Here's how the part is built. I have some questions about the finished solid (model axes, mm). A direction names the side the tool comes from. Round coordinates to 2 decimals unless told otherwise and drop trailing zeros. Order: outer loops, then holes, each group sorted by start corner. A loop starts at its lowest first (then second) coordinate and runs counter-clockwise, first axis right, second up. Notation, with made-up numbers: (-38.5, 76) -> (-13.5, 76) arc R16 ccw to (-13.5, 82) -> close; hole circle Ø11 at (24.5, 50). An arc over 180 degrees is marked (long way). Use a Markdown table: item, result. Add a question column.
from build123d import *

# Parameters (mm, degrees)
SKETCH1_W           = 8.25
SKETCH1_H           = 2.1
SKETCH1_H_2         = 20.8
SKETCH1_R           = 2.275
BOSS_EXTRUDE1_DEPTH = 28.45
BOSS_EXTRUDE2_START = -28.45
SKETCH1_4_W         = 8.25
SKETCH1_4_H         = 2.1
SKETCH1_4_H_2       = 20.8
SKETCH1_4_R         = 2.275
SKETCH1_4_W_2       = 40.9
SKETCH1_4_W_3       = 0.2
SKETCH1_4_W_4       = 8.45
SKETCH1_4_R_2       = 1.7
BOSS_EXTRUDE2_DEPTH = 2
SKETCH1_5_W         = 69.95
SKETCH1_5_H         = 38
BOSS_EXTRUDE3_DEPTH = 30.45
SKETCH1_6_W         = 69.95
SKETCH1_6_H         = 38
BOSS_EXTRUDE4_DEPTH = 5


with BuildPart() as part:
    # Sketch1 → Boss-Extrude1 (new body)
    # profile 1 of 5: a face of its own
    with BuildSketch(Plane.XY):
        Polygon((-28.9, 12.5), (-20.65, 12.5), (-9.8, 12.5), (-9.8, 23.6), (-28.9, 23.6), align=None)
    # profile 2 of 5: a face of its own
    with BuildSketch(Plane.XY):
        with Locations((-24.775, 11.45)):
            Rectangle(SKETCH1_W, SKETCH1_H)
    # profile 3 of 5: a face of its own
    with BuildSketch(Plane.XY):
        with Locations((-24.775, 0)):
            Rectangle(SKETCH1_W, SKETCH1_H_2)
        with Locations((-24.55, -4.85)):
            Circle(SKETCH1_R, mode=Mode.SUBTRACT)
        with Locations((-24.55, 4.85)):
            Circle(SKETCH1_R, mode=Mode.SUBTRACT)
    # profile 4 of 5: a face of its own
    with BuildSketch(Plane.XY):
        Polygon((9.8, 12.5), (20.45, 12.5), (28.9, 12.5), (37.05, 12.5), (37.05, 23.6), (9.8, 23.6), align=None)
    # profile 5 of 5: a face of its own
    with BuildSketch(Plane.XY):
        Polygon((28.9, 12.5), (28.9, 10.4), (28.9, -10.4), (37.05, -10.4), (37.05, 12.5), align=None)
        with Locations((32.55, -4.85)):
            Circle(SKETCH1_R, mode=Mode.SUBTRACT)
        with Locations((32.55, 4.85)):
            Circle(SKETCH1_R, mode=Mode.SUBTRACT)
    extrude(amount=-BOSS_EXTRUDE1_DEPTH)

    # Sketch1<4> → Boss-Extrude2 (add)
    # profile 1 of 16: a face of its own
    with BuildSketch(Plane.XY.offset(BOSS_EXTRUDE2_START)):
        Polygon((-28.9, 12.5), (-20.65, 12.5), (-9.8, 12.5), (-9.8, 23.6), (-28.9, 23.6), align=None)
    # profile 2 of 16: a face of its own
    with BuildSketch(Plane.XY.offset(BOSS_EXTRUDE2_START)):
        Polygon((9.8, 12.5), (20.45, 12.5), (28.9, 12.5), (37.05, 12.5), (37.05, 23.6), (9.8, 23.6), align=None)
    # profile 3 of 16: a face of its own
    with BuildSketch(Plane.XY.offset(BOSS_EXTRUDE2_START)):
        Polygon((-20.65, 10.4), (-20.45, 10.4), (20.45, 10.4), (20.45, 12.5), (9.8, 12.5), (-9.8, 12.5), (-20.65, 12.5), align=None)
    # profile 4 of 16: a face of its own
    with BuildSketch(Plane.XY.offset(BOSS_EXTRUDE2_START)):
        with Locations((-24.775, 11.45)):
            Rectangle(SKETCH1_4_W, SKETCH1_4_H)
    # profile 5 of 16: a face of its own
    with BuildSketch(Plane.XY.offset(BOSS_EXTRUDE2_START)):
        with Locations((-24.775, 0)):
            Rectangle(SKETCH1_4_W, SKETCH1_4_H_2)
        with Locations((-24.55, -4.85)):
            Circle(SKETCH1_4_R, mode=Mode.SUBTRACT)
        with Locations((-24.55, 4.85)):
            Circle(SKETCH1_4_R, mode=Mode.SUBTRACT)
    # profile 6 of 16: a face of its own
    with BuildSketch(Plane.XY.offset(BOSS_EXTRUDE2_START)):
        with Locations((-24.55, 4.85)):
            Circle(SKETCH1_4_R)
    # profile 7 of 16: a face of its own
    with BuildSketch(Plane.XY.offset(BOSS_EXTRUDE2_START)):
        with Locations((-24.55, -4.85)):
            Circle(SKETCH1_4_R)
    # profile 8 of 16: a face of its own
    with BuildSketch(Plane.XY.offset(BOSS_EXTRUDE2_START)):
        Rectangle(SKETCH1_4_W_2, SKETCH1_4_H_2)
    # profile 9 of 16: a face of its own
    with BuildSketch(Plane.XY.offset(BOSS_EXTRUDE2_START)):
        with Locations((-20.55, 0)):
            Rectangle(SKETCH1_4_W_3, SKETCH1_4_H_2)
    # profile 10 of 16: a face of its own
    with BuildSketch(Plane.XY.offset(BOSS_EXTRUDE2_START)):
        with Locations((24.675, 0)):
            Rectangle(SKETCH1_4_W_4, SKETCH1_4_H_2)
        with Locations((24.55, -4.85)):
            Circle(SKETCH1_4_R_2, mode=Mode.SUBTRACT)
        with Locations((24.55, 4.85)):
            Circle(SKETCH1_4_R_2, mode=Mode.SUBTRACT)
    # profile 11 of 16: a face of its own
    with BuildSketch(Plane.XY.offset(BOSS_EXTRUDE2_START)):
        with Locations((24.55, 4.85)):
            Circle(SKETCH1_4_R_2)
    # profile 12 of 16: a face of its own
    with BuildSketch(Plane.XY.offset(BOSS_EXTRUDE2_START)):
        with Locations((24.55, -4.85)):
            Circle(SKETCH1_4_R_2)
    # profile 13 of 16: a face of its own
    with BuildSketch(Plane.XY.offset(BOSS_EXTRUDE2_START)):
        with Locations((24.675, 11.45)):
            Rectangle(SKETCH1_4_W_4, SKETCH1_4_H)
    # profile 14 of 16: a face of its own
    with BuildSketch(Plane.XY.offset(BOSS_EXTRUDE2_START)):
        Polygon((28.9, 12.5), (28.9, 10.4), (28.9, -10.4), (37.05, -10.4), (37.05, 12.5), align=None)
        with Locations((32.55, -4.85)):
            Circle(SKETCH1_4_R, mode=Mode.SUBTRACT)
        with Locations((32.55, 4.85)):
            Circle(SKETCH1_4_R, mode=Mode.SUBTRACT)
    # profile 15 of 16: a face of its own
    with BuildSketch(Plane.XY.offset(BOSS_EXTRUDE2_START)):
        with Locations((32.55, 4.85)):
            Circle(SKETCH1_4_R)
    # profile 16 of 16: a face of its own
    with BuildSketch(Plane.XY.offset(BOSS_EXTRUDE2_START)):
        with Locations((32.55, -4.85)):
            Circle(SKETCH1_4_R)
    extrude(amount=-BOSS_EXTRUDE2_DEPTH)

    # Sketch1<5> → Boss-Extrude3 (add)
    with BuildSketch(Plane.XY):
        with Locations((4.075, 6.6)):
            Rectangle(SKETCH1_5_W, SKETCH1_5_H)
        Polygon((37.05, 23.6), (9.8, 23.6), (-9.8, 23.6), (-28.9, 23.6), (-28.9, 12.5), (-28.9, 10.4), (-28.9, -10.4), (28.9, -10.4), (37.05, -10.4), (37.05, 12.5), align=None, mode=Mode.SUBTRACT)
    extrude(amount=-BOSS_EXTRUDE3_DEPTH)

    # Sketch1<6> → Boss-Extrude4 (add)
    with BuildSketch(Plane.XY):
        with Locations((4.075, 6.6)):
            Rectangle(SKETCH1_6_W, SKETCH1_6_H)
        Polygon((37.05, 23.6), (9.8, 23.6), (-9.8, 23.6), (-28.9, 23.6), (-28.9, 12.5), (-28.9, 10.4), (-28.9, -10.4), (28.9, -10.4), (37.05, -10.4), (37.05, 12.5), align=None, mode=Mode.SUBTRACT)
    extrude(amount=BOSS_EXTRUDE4_DEPTH)


solid = part.part
(1) On a 3-axis mill with a long thin cutter (end or side, diameter ignored), from which of +Z, -Z, +X, -X, +Y, -Y can I reach the whole of each face in a straight line? I mean faces 4 (the flat face through (-9.8, 18, -15)), 5 (the flat face through (4, -12.4, -13)), 6 (the flat face through (-20.65, 1, -14)). Say none if no direction works.
(2) If we mould it in two halves opening along X, with no side actions, what happens to faces 1 (the flat face through (37.05, 7, 2)), 2 (the cylindrical face through (-22.38, 5.53, -14.03)), 3 (the flat face through (1, -12, 5))? For each: pulls with the +X half, pulls with the -X half, needs draft (parallel to the pull), parting line crosses it, or undercut.
(3) I want a section at A-A on y = 20. List the corners of the cut face in (x, z) for me, and give its area (3 significant figures).
(4) Please list where these lines run through material, in increasing order: probe 1 along Y at (x, z) = (-24.5, -16); probe 2 along Y at (x, z) = (4, -2); probe 3 along X at (y, z) = (22, -14). Write a range as from..to.
(5) I want a section at D-D on z = 2. List the corners of the cut face in (x, y) for me, and give its area (3 significant figures).
(6) I want a section at B-B on x = -3. List the corners of the cut face in (y, z) for me, and give its area (3 significant figures).
(7) I want a section at C-C on z = -23.5. List the corners of the cut face in (x, y) for me (3 decimals).
(8) I'm going to push flat-ended pins straight in: P1, Ø3, axis at x = 32, y = 7.5, coming from the +Z side; P2, Ø1.4, axis at x = -25.5, y = -4, coming from the +Z side. Where does each tip first touch, or does it pass through?
Output:
| question | item | result |
|---|---|---|
| 1 | face 4 | +Z, -Z |
| 1 | face 5 | +Z, -Z, +X, -X, -Y |
| 1 | face 6 | +Z |
| 2 | face 1 | undercut |
| 2 | face 2 | undercut |
| 2 | face 3 | needs draft |
| 3 | outline | (-30.9, -30.45) -> (-9.8, -30.45) -> (-9.8, 0) -> (-28.9, 0) -> (-28.9, 5) -> (-30.9, 5) -> close; (9.8, -30.45) -> (39.05, -30.45) -> (39.05, 5) -> (37.05, 5) -> (37.05, 0) -> (9.8, 0) -> close |
| 3 | area | 1,550 mm² |
| 4 | probe 1 | -12.4..-7.12, -2.58..2.58, 7.12..25.6 |
| 4 | probe 2 | -12.4..-10.4, 23.6..25.6 |
| 4 | probe 3 | -30.9..-9.8, 9.8..39.05 |
| 5 | outline | (-30.9, -12.4) -> (39.05, -12.4) -> (39.05, 25.6) -> (-30.9, 25.6) -> close; hole (-28.9, -10.4) -> (37.05, -10.4) -> (37.05, 23.6) -> (-28.9, 23.6) -> close |
| 5 | area | 416 mm² |
| 6 | outline | (-12.4, -30.45) -> (12.5, -30.45) -> (12.5, -28.45) -> (-10.4, -28.45) -> (-10.4, 5) -> (-12.4, 5) -> close; (23.6, -30.45) -> (25.6, -30.45) -> (25.6, 5) -> (23.6, 5) -> close |
| 6 | area | 188 mm² |
| 7 | outline | (-30.9, -12.4) -> (39.05, -12.4) -> (39.05, 25.6) -> (-30.9, 25.6) -> close; hole circle Ø4.55 at (-24.55, -4.85); hole circle Ø4.55 at (-24.55, 4.85); hole (-20.65, -10.4) -> (28.9, -10.4) -> (28.9, 12.5) -> (9.8, 12.5) -> (9.8, 23.6) -> (-9.8, 23.6) -> (-9.8, 12.5) -> (-20.65, 12.5) -> close; hole circle Ø4.55 at (32.55, -4.85); hole circle Ø4.55 at (32.55, 4.85) |
| 8 | P1 | z = 0 |
| 8 | P2 | z = -28.45 |
